Read the model definition and answer for the solid it produces. Units are mm, in the model's axes. Face numbers are marked on the shaded views. Coordinates: 2 decimals unless noted, no trailing zeros. Write each loop counter-clockwise with the first axis right and the second up, starting at its lowest first coordinate (ties: lowest second). Pieces come first, ordered by that corner, then holes.
1) Determine the mould class of the marked faces 1, 2 and 3 for opening direction Y: +Y half, -Y half, draft (parallel to the pull), parting line (faces both ways), or undercut.
2) The part is cut by section A-A (x = -2.5). Determine the outline of the cut face in (y, z), then the cut area to 3 significant figures.
3) The part is cut by section C-C (z = 165). Determine the outline of the cut face in (x, y).
4) Find the intervals of material crossed by line 1 (Y direction, x = 8.25, z = 179.5); line 2 (Y direction, x = -10.5, z = 42), in increasing order.
5) This flat-tipped pin is pushed along its axis until it touches: pin 1 Ø5 at (y, z) = (12, 80.5) entering from +X. Where does it stop, or does it pass through?
Autodesk Inventor part; units mm, degrees
ref_plane "Start Plane" through (0, 0, 15) normal (0, 0, 1) x (1, 0, 0)
ref_plane "End Plane" through (0, 0, 215) normal (0, 0, 1) x (1, 0, 0)
ref_plane "Work Plane4" through (678.5, -9, 215) normal (0, 0, 1) x (1, 0, 0)
ref_plane "Start Plane" through (0, 0, 15) normal (0, 0, 1) x (1, 0, 0)
ref_plane "End Plane" through (0, 0, 215) normal (0, 0, 1) x (1, 0, 0)
sketch "Sketch" plane through (0, 0, 0) normal (0, 0, 1) x (1, 0, 0)
  line L0 (-15, -9) -> (-15, 9)
  line L1 (-9, 15) -> (9, 15)
  line L2 (15, 9) -> (15, -9)
  line L3 (9, -15) -> (-9, -15)
  arc A0 (-15, -9) -> (-9, -15) centre (-9, -9) ccw
  arc A1 (-9, 15) -> (-15, 9) centre (-9, 9) ccw
  arc A2 (15, 9) -> (9, 15) centre (9, 9) ccw
  arc A3 (9, -15) -> (15, -9) centre (9, -9) ccw
  arc A4 (-9, 12) -> (-12, 9) centre (-9, 9) ccw
  line L4 (-9, 12) -> (9, 12)
  arc A5 (12, 9) -> (9, 12) centre (9, 9) ccw
  line L5 (12, 9) -> (12, -9)
  arc A6 (9, -12) -> (12, -9) centre (9, -9) ccw
  line L6 (9, -12) -> (-9, -12)
  arc A7 (-12, -9) -> (-9, -12) centre (-9, -9) ccw
  line L7 (-12, -9) -> (-12, 9)
  line L8 (0, 22.7397) -> (0, -22.7397) construction
  line L9 (-22.7397, 0) -> (22.7397, 0) construction
  dimension "d7" = 6
  dimension "d10" = 30
  dimension "d11" = 30
  dimension "d12" = 3
  dimension "d15" = 15
  dimension "d16" = 15
extrude "Body" add sketch "Sketch" along normal up to surface (200 mm away) from surface at 15
sketch "Sketch3" plane through (0, 0, 0) normal (0, 0, 1) x (1, 0, 0)
  line L0 (0, 0) -> (10, 0)
ref_plane "Work Plane3" through (0, 0, 0) normal (0, -1, 0) x (1, 0, 0)
ref_plane "Work Plane4" through (678.5, -9, 215) normal (0, 0, 1) x (1, 0, 0)
split "Split1" plane through (678.5, -9, 215) removes the side toward (0, 0, 1)
ref_plane "Work Plane5" through (-521.5, -9, 15) normal (0, 0, -1) x (-1, 0, 0)
split "Split2" plane through (-521.5, -9, 15) removes the side toward (0, 0, -1)
sketch "Sketch4" plane through (0, 0, 0) normal (0, -1, 0) x (1, 0, 0)
  line L0 (-2, 15) -> (12, 15)
  line L1 (-2, 215) -> (12, 215)
  dimension "d18" = 200
equation "\"d7\" = G_IR"
equation "\"d10\" = G_H"
equation "\"d11\" = G_W"
equation "\"d12\" = G_T"
equation "\"d15\" = 0.5 * d10"
equation "\"d16\" = 0.5 * d11"
equation "\"d3\" = G_L"
equation "\"G_W\" = 30"
equation "\"G_H\" = 30"
equation "\"G_T\" = 3"
equation "\"G_IR\" = 6"
equation "\"G_L\" = d18"
equation "\"G_OFFSET_START\" = -15"
equation "\"G_OFFSET_END\" = -15"
equation "\"d13\" = -G_OFFSET_START"
equation "\"d14\" = G_OFFSET_END + B_L"
properties part number "DIN EN 10219-2 - 30 x 30 x 3  - 200" material "Steel, Mild"
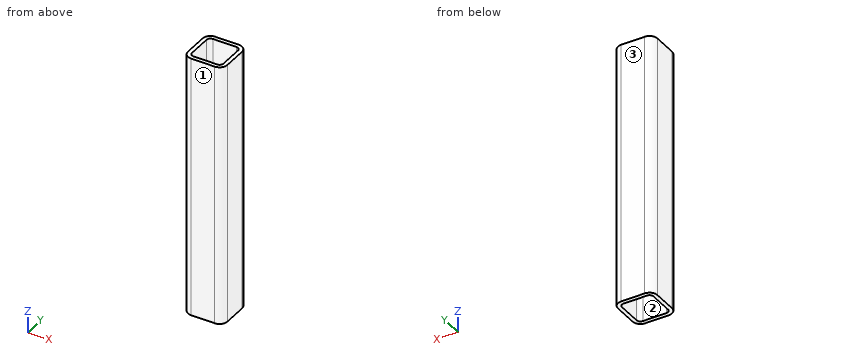
Reported:
1. face 1: -Y half
1. face 2: undercut
1. face 3: +Y half
2. outline: (-15, 15) - (-12, 15) - (-12, 215) - (-15, 215) - close; (12, 15) - (15, 15) - (15, 215) - (12, 215) - close
2. area: 1,200 mm2
3. outline: (-15, -9) arc R6 ccw to (-9, -15) - (9, -15) arc R6 ccw to (15, -9) - (15, 9) arc R6 ccw to (9, 15) - (-9, 15) arc R6 ccw to (-15, 9) - close; hole (-12, -9) arc R3 ccw to (-9, -12) - (9, -12) arc R3 ccw to (12, -9) - (12, 9) arc R3 ccw to (9, 12) - (-9, 12) arc R3 ccw to (-12, 9) - close
4. line 1: y = -15 to -12, 12 to 15
4. line 2: y = -14.81 to -11.6, 11.6 to 14.81
5. pin 1: stops at x = 14.98
